```python
from build123d import *

# Parameters (mm, degrees)
SKETCH1_R               = 35
BOSS_EXTRUDE1_DEPTH     = 15
SKETCH2_R               = 3
CUT_EXTRUDE1_DEPTH      = 52.720402164
CUT_EXTRUDE3_DEPTH      = 52.720402164
CIRPATTERN1_COUNT       = 5
FILLET4_R               = 2.2
FILLET5_R               = 3.2
SKETCH5_R               = 36.5
SKETCH5_R_2             = 35
BOSS_EXTRUDE2_DEPTH     = 1
BOSS_EXTRUDE3_START     = -1
SKETCH6_R               = 36.5
SKETCH6_R_2             = 35
BOSS_EXTRUDE3_DEPTH     = 1
SKETCH7_R               = 1.55
CUT_EXTRUDE4_DEPTH      = 54.754069613
CUT_EXTRUDE5_DEPTH      = 54.754069641
CUT_EXTRUDE5_DEPTH_BACK = 1
CUT_EXTRUDE5_START      = 20
SKETCH8_R               = 3


with BuildPart() as part:
    # Sketch1 → Boss-Extrude1 (new body)
    with BuildSketch(Plane.XY):
        Circle(SKETCH1_R)
    extrude(amount=BOSS_EXTRUDE1_DEPTH)

    # Sketch2 → Cut-Extrude1 (cut, through all)
    with BuildSketch(Plane(origin=(0, 0, 0), x_dir=(-1, 0, 0), z_dir=(0, 0, -1))):
        Circle(SKETCH2_R)
    extrude(amount=-CUT_EXTRUDE1_DEPTH, mode=Mode.SUBTRACT)

    # Sketch4 → Cut-Extrude3 (cut, through all)
    with BuildSketch(Plane(origin=(0, 0, 0), x_dir=(-1, 0, 0), z_dir=(0, 0, -1))):
        with BuildLine():
            Line((2.104758878, 5.081337429), (12.437211552, 30.026084807))
            ThreePointArc((12.437211552, 30.026084807), (0, 32.5), (-12.437211552, 30.026084807))
            Line((-12.437211552, 30.026084807), (-2.104758878, 5.081337429))
            ThreePointArc((-2.104758878, 5.081337429), (0, 5.5), (2.104758878, 5.081337429))
        make_face()
    cut_extrude3 = extrude(amount=-CUT_EXTRUDE3_DEPTH, mode=Mode.SUBTRACT)

    # CirPattern1: Cut-Extrude3 ×5 about axis
    cirpattern1_axis = Axis((0, 0, 0), (0, 0, 1))
    for i in range(1, CIRPATTERN1_COUNT):
        add(cut_extrude3.rotate(cirpattern1_axis, i * 360 / CIRPATTERN1_COUNT), mode=Mode.SUBTRACT)

    # Fillet4
    fillet4_edges = [part.edges().sort_by_distance(p)[0] for p in [
        (-2.104758878, 5.081337429, 7.5),
        (2.104758878, 5.081337429, 7.5),
        (-5.483045336, -0.431525027, 7.5),
        (-4.182232811, 3.571964266, 7.5),
        (-1.283949501, -5.348034562, 7.5),
        (-4.689520904, -2.873742106, 7.5),
        (4.689520904, -2.873742106, 7.5),
        (1.283949501, -5.348034562, 7.5),
        (4.182232811, 3.571964266, 7.5),
        (5.483045336, -0.431525027, 7.5),
    ]]
    fillet(fillet4_edges, radius=FILLET4_R)

    # Fillet5
    fillet5_edges = [part.edges().sort_by_distance(p)[0] for p in [
        (12.437211552, 30.026084807, 7.5),
        (-12.437211552, 30.026084807, 7.5),
        (-24.713193882, 21.107061571, 7.5),
        (-32.399813346, -2.549920611, 7.5),
        (-27.710805342, -16.981203353, 7.5),
        (-7.586974325, -31.602022413, 7.5),
        (7.586974325, -31.602022413, 7.5),
        (27.710805342, -16.981203353, 7.5),
        (32.399813346, -2.549920611, 7.5),
        (24.713193882, 21.107061571, 7.5),
    ]]
    fillet(fillet5_edges, radius=FILLET5_R)

    # Sketch5 → Boss-Extrude2 (add)
    with BuildSketch(Plane(origin=(0, 0, 0), x_dir=(-1, 0, 0), z_dir=(0, 0, -1))):
        Circle(SKETCH5_R)
        Circle(SKETCH5_R_2, mode=Mode.SUBTRACT)
    extrude(amount=-BOSS_EXTRUDE2_DEPTH)

    # Sketch6 → Boss-Extrude3 (add)
    with BuildSketch(Plane.XY.offset(15).offset(BOSS_EXTRUDE3_START)):
        with Locations(Location((0, 0, 0), (0, 0, 180))):
            Circle(SKETCH6_R)
        with Locations(Location((0, 0, 0), (0, 0, 180))):
            Circle(SKETCH6_R_2, mode=Mode.SUBTRACT)
    extrude(amount=BOSS_EXTRUDE3_DEPTH)

    # Sketch7 → Cut-Extrude4 (cut, through all)
    with BuildSketch(Plane(origin=(0, 0, 0), x_dir=(1, 0, 0), z_dir=(0, 1, 0))):
        with Locations(Location((0, -7.5, 0), (0, 0, 90))):
            Circle(SKETCH7_R)
    extrude(amount=CUT_EXTRUDE4_DEPTH, mode=Mode.SUBTRACT)

    # Sketch8 → Cut-Extrude5 (cut, two sides: drawn at the far end of the back side and taken through both)
    with BuildSketch(Plane(origin=(0, 0, 0), x_dir=(1, 0, 0), z_dir=(0, 1, 0)).offset(CUT_EXTRUDE5_START - CUT_EXTRUDE5_DEPTH_BACK)):
        with Locations(Location((0, -7.5, 0), (0, 0, 90))):
            Circle(SKETCH8_R)
    extrude(amount=CUT_EXTRUDE5_DEPTH + CUT_EXTRUDE5_DEPTH_BACK, mode=Mode.SUBTRACT)


solid = part.part
```
Read the model definition and answer for the solid it produces. Units are mm, in the model's axes. A direction names the side the tool comes from. Coordinates: 2 decimals unless noted, no trailing zeros. Loops run counter-clockwise (first coordinate to the right, second up) from the corner with the lowest first, then second, coordinate; pieces in that order, holes last. Notation, with made-up numbers: (-2, -3.5) -> (50, -3.5) arc R20 cw to (50, 15.5) -> close; hole circle Ø3 at (16.25, 18). An arc over 180 degrees is marked (long way). Return JSON: item names as keys, results as strings.
Item 1: Find section A-A (y = 30). Determine the outline of the cut face in (x, z), plus the area to 3 significant figures.
Answers:
{"outline": "(-20.79, 0) -> (-10.79, 0) -> (-10.79, 15) -> (-20.79, 15) -> (-20.79, 14) -> (-18.03, 14) -> (-18.03, 1) -> (-20.79, 1) -> close; (10.79, 0) -> (20.79, 0) -> (20.79, 1) -> (18.03, 1) -> (18.03, 14) -> (20.79, 14) -> (20.79, 15) -> (10.79, 15) -> close", "area": "228 mm2"}
Item 2: Find section B-B (x = -12.5). Determine the outline of the cut face in (y, z), plus the area to 3 significant figures.
Answers:
{"outline": "(-34.29, 0) -> (-30, 0) -> (-30, 15) -> (-34.29, 15) -> (-34.29, 14) -> (-32.69, 14) -> (-32.69, 1) -> (-34.29, 1) -> close; (-7.66, 0) -> (-0.98, 0) -> (-0.98, 15) -> (-7.66, 15) -> close; (10.68, 0) -> (34.29, 0) -> (34.29, 1) -> (32.69, 1) -> (32.69, 14) -> (34.29, 14) -> (34.29, 15) -> (10.68, 15) -> close", "area": "477 mm2"}
Item 3: Find section C-C (x = 30.5). Determine the outline of the cut face in (y, z).
Answers:
{"outline": "(-20.05, 0) -> (-2.06, 0) -> (-2.06, 15) -> (-20.05, 15) -> (-20.05, 14) -> (-17.17, 14) -> (-17.17, 1) -> (-20.05, 1) -> close; (11.22, 0) -> (20.05, 0) -> (20.05, 1) -> (17.17, 1) -> (17.17, 14) -> (20.05, 14) -> (20.05, 15) -> (11.22, 15) -> close"}
Item 4: Flat-ended cylindrical pins translate along their axes: P1, Ø5, axis at x = -22, z = 11, coming from the +Y side; P2, Ø6, axis at x = -16.5, y = -11, coming from the +Z side; P3, Ø8, axis at x = -1, z = 3.5, coming from the -Y side; P4, Ø8, axis at x = -12.5, z = 6.5, coming from the -Y side. Find the tip coordinate at first contact, or state that the pin passes through.
Answers:
{"P1": "stops at y = 29.06", "P2": "stops at z = 15", "P3": "stops at y = -36.5", "P4": "stops at y = -33.95"}
Item 5: Find the intervals of material crossed by probe 1 along X at (y, z) = (3.5, 3.5); probe 2 along Y at (x, z) = (-8.5, 10.5); probe 3 along Y at (x, z) = (-24.5, 14.25), in increasing order.
Answers:
{"probe 1": "x = -34.82 to -32.31, -4.87 to 4.87, 32.31 to 34.82", "probe 2": "y = -33.95 to -30.45, -5.21 to -0.67, 7.26 to 20.52, 31.37 to 33.95", "probe 3": "y = -27.06 to -21.35, -15.01 to -1.93, 19.67 to 27.06"}
Item 6: For a pull along Z with two mould halves and no side action, classify faces 1 (the cylindrical face through (2.662, 33.661, 6.116)), 2 (the flat face through (1, -8, 0)), 3 (the cylindrical face through (4.89, 3.59, 7.6)) as +Z half, -Z half, draft (parallel to the pull), parting line (faces both ways), or undercut.
Answers:
{"face 1": "undercut", "face 2": "-Z half", "face 3": "draft"}
Item 7: Find section D-D (z = 12.5). Count the separate pieces of the cut face and the enclosed holes in it, plus the area to 3 significant figures.
Answers:
{"separate pieces": "1", "enclosed holes": "6", "area": "1,840 mm2"}
Item 8: For faces 4 (the cylindrical face through (-28, -21, 7)), 5 (the cylindrical face through (1.848, -5.777, 7.605)), determine the directions among +Z, -Z, +X, -X, +Y, -Y from which every point of the face is accessible in a straight line to the end or side of a thin tool.
Answers:
{"face 4": "none", "face 5": "+Z, -Z"}
